from build123d import *

# Parameters (mm, degrees)
BOSS_EXTRUDE1_DEPTH = 5.588
FILLET1_R           = 19.05
SKETCH2_R           = 1.5
SKETCH2_R_2         = 3.75
CUT_EXTRUDE1_DEPTH  = 438.386266067


with BuildPart() as part:
    # Sketch1 → Boss-Extrude1 (new body)
    with BuildSketch(Plane(origin=(0, 0, 0), x_dir=(1, 0, 0), z_dir=(0, 1, 0))):
        Polygon((0, 161.6), (0, 0), (63.5, 0), (63.5, 31.75), (55.88, 31.75), (55.88, 26.67), (45.72, 26.67), (45.72, 41.91), (55.88, 41.91), (55.88, 36.83), (63.5, 36.83), (63.5, 50.8), (342.9, 50.8), (342.9, 36.83), (350.52, 36.83), (350.52, 41.91), (360.68, 41.91), (360.68, 26.67), (350.52, 26.67), (350.52, 31.75), (342.9, 31.75), (342.9, 0), (406.4, 0), (406.4, 161.6), (342.9, 161.6), (342.9, 110.8), (63.5, 110.8), (63.5, 161.6), align=None)
    extrude(amount=BOSS_EXTRUDE1_DEPTH)

    # Fillet1
    fillet1_edges = [part.edges().sort_by_distance(p)[0] for p in [
        (63.5, 2.794, 0),
        (63.5, 2.794, -161.6),
        (342.9, 2.794, -161.6),
        (342.9, 2.794, 0),
    ]]
    fillet(fillet1_edges, radius=FILLET1_R)

    # Sketch2 → Cut-Extrude1 (cut, through all)
    with BuildSketch(Plane(origin=(0, 5.588, 0), x_dir=(1, 0, 0), z_dir=(0, 1, 0))):
        with Locations(Location((366.4, 80.8, 0), (0, 0, 270))):
            Circle(SKETCH2_R)
        with Locations(Location((386.4, 80.8, 0), (0, 0, 270))):
            Circle(SKETCH2_R)
        with Locations(Location((366.4, 103.3, 0), (0, 0, 270))):
            Circle(SKETCH2_R_2)
        with Locations(Location((386.4, 103.3, 0), (0, 0, 270))):
            Circle(SKETCH2_R_2)
        with Locations(Location((386.4, 58.3, 0), (0, 0, 90))):
            Circle(SKETCH2_R_2)
        with Locations(Location((366.4, 58.3, 0), (0, 0, 90))):
            Circle(SKETCH2_R_2)
        with Locations(Location((306.4, 103.3, 0), (0, 0, 270))):
            Circle(SKETCH2_R_2)
        with Locations(Location((326.4, 103.3, 0), (0, 0, 270))):
            Circle(SKETCH2_R_2)
        with Locations(Location((326.4, 80.8, 0), (0, 0, 270))):
            Circle(SKETCH2_R)
        with Locations(Location((306.4, 80.8, 0), (0, 0, 270))):
            Circle(SKETCH2_R)
        with Locations(Location((306.4, 58.3, 0), (0, 0, 90))):
            Circle(SKETCH2_R_2)
        with Locations(Location((326.4, 58.3, 0), (0, 0, 90))):
            Circle(SKETCH2_R_2)
    extrude(amount=-CUT_EXTRUDE1_DEPTH, mode=Mode.SUBTRACT)


solid = part.part
Model file for the job. Use its own axes, mm. A direction names the side the tool comes from. Coordinates: 2 decimals unless noted, no trailing zeros. Order: outer loops, then holes, each group sorted by start corner. A loop starts at its lowest first (then second) coordinate and runs counter-clockwise, first axis right, second up. Notation, with made-up numbers: M -7,15.25 L -1,15.25 A23 cw -1,54.25 Z; hole C 83,56.5 d9. An arc over 180 degrees is marked long. Return JSON: item names as keys, results as strings.
1. Saw through at D-D (x = 211). Give the cut face in (y, z).
Ans:
{"outline": "M 0,-110.8 L 5.59,-110.8 L 5.59,-50.8 L 0,-50.8 Z"}
2. Saw through at C-C (y = 2.05). Give the number of separate pieces and of enclosed holes in the cut face, and give its area (3 significant figures).
Ans:
{"separate pieces": "1", "enclosed holes": "12", "area": "36,200 mm^2"}
3. Saw through at A-A (z = -133). Give the cut face in (x, y).
Ans:
{"outline": "M 0,0 L 63.5,0 L 63.5,5.59 L 0,5.59 Z; M 342.9,0 L 406.4,0 L 406.4,5.59 L 342.9,5.59 Z"}
4. Flat gauge pins, fed straight in: pin 1 (3 mm diameter, centred on x = 179, y = 3, fed in from +Z); pin 2 (3 mm diameter, centred on x = 52, y = 1.5, fed in from +Z); pin 3 (3 mm diameter, centred on x = 58, y = 3.5, fed in from -Z). Where does each tip first touch, or does it go through?
Ans:
{"pin 1": "z = -50.8", "pin 2": "z = -0.99", "pin 3": "z = -157.3"}
5. Saw through at B-B (z = -58.3). Give the cut face in (x, y).
Ans:
{"outline": "M 0,0 L 302.65,0 L 302.65,5.59 L 0,5.59 Z; M 310.15,0 L 322.65,0 L 322.65,5.59 L 310.15,5.59 Z; M 330.15,0 L 362.65,0 L 362.65,5.59 L 330.15,5.59 Z; M 370.15,0 L 382.65,0 L 382.65,5.59 L 370.15,5.59 Z; M 390.15,0 L 406.4,0 L 406.4,5.59 L 390.15,5.59 Z"}
6. Drill centre lines: probe 1 along Z at (x, y) = (386.4, 4.5); probe 2 along X at (y, z) = (1.2, -58.3); probe 3 along X at (y, z) = (1.25, -80.8). Where is each one in solid material? Low to high.
Ans:
{"probe 1": "-161.6 to -107.05, -99.55 to -82.3, -79.3 to -62.05, -54.55 to 0", "probe 2": "0 to 302.65, 310.15 to 322.65, 330.15 to 362.65, 370.15 to 382.65, 390.15 to 406.4", "probe 3": "0 to 304.9, 307.9 to 324.9, 327.9 to 364.9, 367.9 to 384.9, 387.9 to 406.4"}
7. Pull direction X, two halves, no side cores. Call faces 4 (the face through (329.56, 2.83, -101.28)), 5 (the face through (200, 5.588, -82)): +X half, -X half, draft (parallel to the pull), parting line (faces both ways), or undercut.
Ans:
{"face 4": "undercut", "face 5": "draft"}
8. Tool access for faces 1 (the face through (369.56, 2.83, -101.28)), 2 (the face through (58.07, 2.83, -155.87)), 3 (the face through (348.33, 2.83, -5.73)): list every direction of +Z, -Z, +X, -X, +Y, -Y with a clear straight run to the whole face (end or side of a thin tool).
Ans:
{"face 1": "+Y, -Y", "face 2": "-Z, +Y, -Y", "face 3": "+Z, +Y, -Y"}
